from build123d import *

# Parameters (mm, degrees)
BOX_W     = 40
BOX_H     = 40
BOX_DEPTH = 3
FILLET_R  = 1


with BuildPart() as cone001:
    # Cone001 → Cone001 (revolve)
    with BuildSketch(Plane(origin=(20, 20, 0), x_dir=(1, 0, 0), z_dir=(0, -1, 0))):
        Polygon((0, 0), (15, 0), (3, 43), (0, 43), align=None)
    revolve(axis=Axis((20, 20, 0), (0, 0, 1)))


with BuildPart() as cut:
    # Cone → Cone (revolve)
    with BuildSketch(Plane(origin=(20, 20, 3), x_dir=(1, 0, 0), z_dir=(0, -1, 0))):
        Polygon((0, 0), (16, 0), (4, 40), (0, 40), align=None)
    revolve(axis=Axis((20, 20, 3), (0, 0, 1)))

    # Cut: cut Cone001
    add(cone001.part, mode=Mode.SUBTRACT)


with BuildPart() as cone002:
    # Cone002 → Cone002 (revolve)
    with BuildSketch(Plane(origin=(20, 20, 0), x_dir=(1, 0, 0), z_dir=(0, -1, 0))):
        Polygon((0, 0), (15, 0), (3, 43), (0, 43), align=None)
    revolve(axis=Axis((20, 20, 0), (0, 0, 1)))


with BuildPart() as fusion:
    # Box → Box (new body)
    with BuildSketch(Plane.XY):
        with Locations((20, 20)):
            Rectangle(BOX_W, BOX_H)
    extrude(amount=BOX_DEPTH)

    # Fillet
    fillet_edges = [fusion.edges().sort_by_distance(p)[0] for p in [
        (0, 0, 1.5),
        (0, 40, 1.5),
        (40, 0, 1.5),
        (40, 40, 1.5),
    ]]
    fillet(fillet_edges, radius=FILLET_R)

    # Cut001: cut Cone002
    add(cone002.part, mode=Mode.SUBTRACT)

    # Fusion: union Cut
    add(cut.part)


solid = fusion.part
CAD build for the part. Positions are in the model's coordinates, mm. A direction names the side the tool comes from. Coordinates: 2 decimals unless noted, no trailing zeros. Loops run counter-clockwise (first coordinate to the right, second up) from the corner with the lowest first, then second, coordinate; pieces in that order, holes last. Notation, with made-up numbers: (-8, 6) -> (21, 6) arc R12 cw to (21, 23) -> close; hole circle Ø4 at (22, 88.5). An arc over 180 degrees is marked (long way). One line per item, written item: value.
1. Pull direction X, two halves, no side cores. Call faces 3 (the face through (40, 20, 1)), 4 (the face through (18.067, 11.296, 21.801)), 5 (the face through (21, 23, 43)): pulls with the +X half, pulls with the -X half, needs draft (parallel to the pull), parting line crosses it, or undercut.
Answers:
face 3: pulls with the +X half
face 4: undercut
face 5: needs draft
2. Which spindle directions (+Z, -Z, +X, -X, +Y, -Y) get a long thin tool onto all of the face, cutting with end or side? Do faces 1 (the face through (11, 34, 0)), 2 (the face through (11, 34, 3)). Say none if no direction does.
Answers:
face 1: -Z, +X, -X, +Y, -Y
face 2: +Z
3. Slice it at C-C on z = 27.5. Write the cut outline in (x, y).
Answers:
outline: circle Ø17.3 at (20, 20); hole circle Ø14.65 at (20, 20)
4. Slice it at D-D on z = 15.5. Write the cut outline in (x, y).
Answers:
outline: circle Ø24.5 at (20, 20); hole circle Ø21.35 at (20, 20)
5. Slice it at A-A on x = 20. Write the cut outline in (y, z).
Answers:
outline: (0, 0) -> (5, 0) -> (17, 43) -> (16, 43) -> (4, 3) -> (0, 3) -> close; (23, 43) -> (35, 0) -> (40, 0) -> (40, 3) -> (36, 3) -> (24, 43) -> close
6. Drill centre lines: line 1 (Z direction, x = 3, y = 38.5); line 2 (X direction, y = 18.5, z = 39); line 3 (Y direction, x = 24, z = 7). Where is each one in solid material? Low to high. Write a range as [from, to].
Answers:
line 1: z = [0, 3]
line 2: x = [15.02, 16.17], [23.83, 24.98]
line 3: y = [5.75, 7.58], [32.42, 34.25]
7. Flat gauge pins, fed straight in: P1, Ø12, axis at x = 23, z = 26, coming from the +Y side; P2, Ø4, axis at y = 23.5, z = 24.5, coming from the +X side; P3, Ø8, axis at x = 14.5, z = 27.5, coming from the +Y side. Where does each tip first touch, or does it go through?
Answers:
P1: stops at y = 30.75
P2: stops at x = 29.76
P3: stops at y = 29.12
